Read the model definition and answer for the solid it produces. Units are mm, in the model's axes. A direction names the side the tool comes from. Coordinates: 2 decimals unless noted, no trailing zeros. Loops run counter-clockwise (first coordinate to the right, second up) from the corner with the lowest first, then second, coordinate; pieces in that order, holes last. Notation, with made-up numbers: (-17, -34) - (15, -34) arc R9 ccw to (15, -20) - close; hole circle Ø5 at (83.5, 55). An arc over 180 degrees is marked (long way). Use one line per item in the form item = value. Start each with the question number.
1) Consider line 1 (Y direction, x = 13.5, z = 3); line 2 (Y direction, x = -24.25, z = 2.75); line 3 (X direction, y = -5.5, z = 3.5). Determine where each line is inside the solid, lowest interval first.
2) Each of these flat-tipped pins is pushed along its axis until it touches: P1, Ø8, axis at x = 13.5, y = 0, coming from the -Z side; P2, Ø13, axis at x = -24.25, y = 0, coming from the -Z side; P3, Ø17.5, axis at x = -26.5, y = -3.5, coming from the -Z side. Where does it stop, or does it pass through?
3) A cutting plane is placed at C-C (x = -24.25). Give the vertices of the cut face in (y, z).
4) A cutting plane is placed at A-A (x = 13.5). Give the vertices of the cut face in (y, z), and give its area (3 significant figures).
5) A cutting plane is placed at B-B (y = 0). Give the vertices of the cut face in (x, z), and give its area (3 significant figures).
6) The mould has two halves that part along X. Classify faces 3 (the face through (-48.5, -1, 5)), 4 (the face through (-1, 1, 0)), 5 (the face through (-24, 0, 5)): released by +X, released by -X, zero draft, split by the parting line, or undercut.
7) Which of the six approach directions +Z, -Z, +X, -X, +Y, -Y give full straight-line access (tool end or side, diameter ignored) to faces 1 (the face through (48.5, -1, 5)), 2 (the face through (-34.411, -4.213, 2.465))?
from build123d import *

# Parameters (mm, degrees)
SKETCH1_W           = 97
SKETCH1_H           = 78.5
BOSS_EXTRUDE1_DEPTH = 10
CUT_EXTRUDE1_REACH  = 65.189
SKETCH2_R           = 5
SKETCH3_R           = 11
CUT_EXTRUDE2_DEPTH  = 5


with BuildPart() as part:
    # Sketch1 → Boss-Extrude1 (new body)
    with BuildSketch(Plane.XY):
        Rectangle(SKETCH1_W, SKETCH1_H)
    extrude(amount=BOSS_EXTRUDE1_DEPTH)

    # Sketch2 → Cut-Extrude1 (cut, up to next)
    with BuildSketch(Plane.XY.offset(10), mode=Mode.PRIVATE) as cut_extrude1_sk1:
        with Locations((13.5, 0)):
            Circle(SKETCH2_R)
    cut_extrude1_tool1 = extrude(cut_extrude1_sk1.sketch, amount=-CUT_EXTRUDE1_REACH, mode=Mode.PRIVATE) & part.part
    add(cut_extrude1_tool1.solids().sort_by_distance((13.5, 0, 10))[0], mode=Mode.SUBTRACT)

    # Sketch3 → Cut-Extrude2 (cut)
    with BuildSketch(Plane(origin=(0, 0, 0), x_dir=(-1, 0, 0), z_dir=(0, 0, -1))):
        with Locations((24.25, 0)):
            Circle(SKETCH3_R)
    extrude(amount=-CUT_EXTRUDE2_DEPTH, mode=Mode.SUBTRACT)


solid = part.part
Found:
q1.line_1 = -39.25 to -5, 5 to 39.25
q1.line_2 = -39.25 to -11, 11 to 39.25
q1.line_3 = -48.5 to -33.78, -14.72 to 48.5
q2.P1 = through
q2.P2 = 5
q2.P3 = 0
q3.outline = (-39.25, 0) - (-11, 0) - (-11, 5) - (11, 5) - (11, 0) - (39.25, 0) - (39.25, 10) - (-39.25, 10) - close
q4.outline = (-39.25, 0) - (-5, 0) - (-5, 10) - (-39.25, 10) - close; (5, 0) - (39.25, 0) - (39.25, 10) - (5, 10) - close
q4.area = 685 mm^2
q5.outline = (-48.5, 0) - (-35.25, 0) - (-35.25, 5) - (-13.25, 5) - (-13.25, 0) - (8.5, 0) - (8.5, 10) - (-48.5, 10) - close; (18.5, 0) - (48.5, 0) - (48.5, 10) - (18.5, 10) - close
q5.area = 760 mm^2
q6.face_3 = released by -X
q6.face_4 = zero draft
q6.face_5 = undercut
q7.face_1 = +Z, -Z, +X, +Y, -Y
q7.face_2 = -Z
